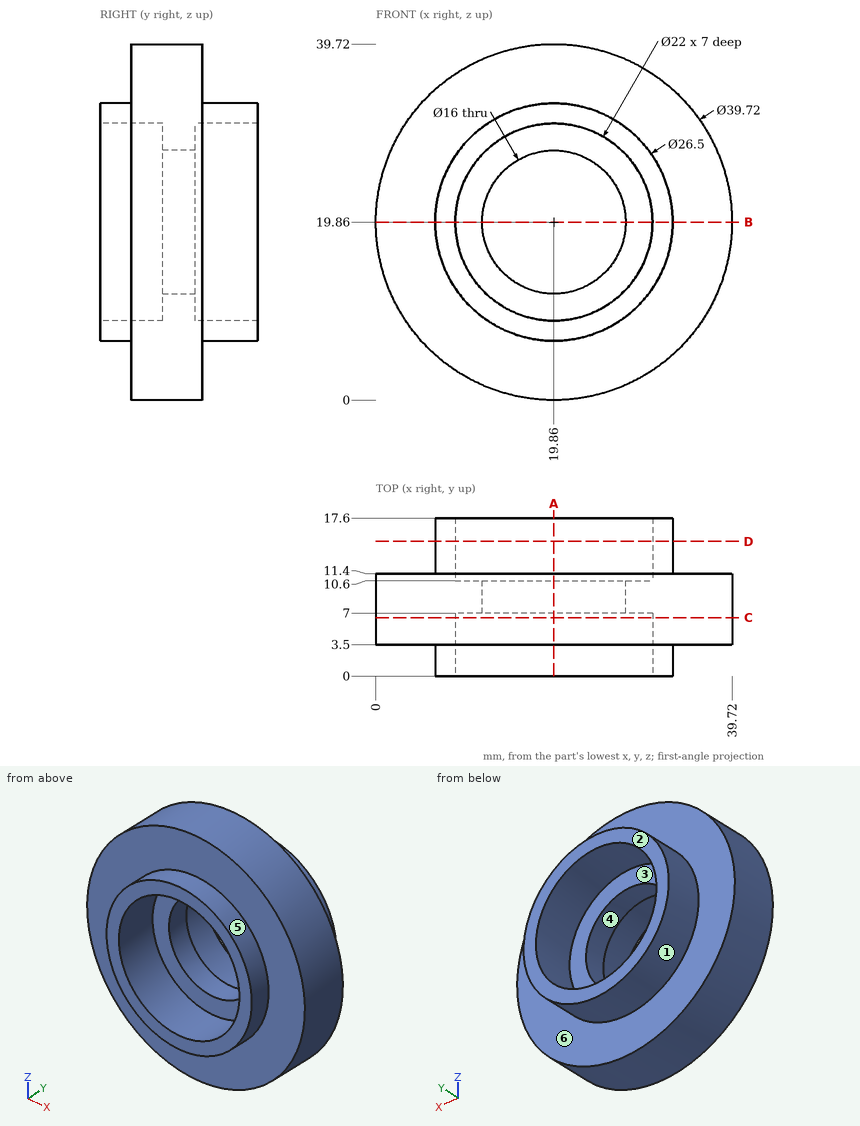
Part print with two shaded views. Sizes in mm from the minimum x, y, z corner. A direction names the side the tool comes from. Coordinates: 2 decimals unless noted, no trailing zeros. Write each loop counter-clockwise with the first axis right and the second up, starting at its lowest first coordinate (ties: lowest second). Pieces come first, ordered by that corner, then holes. Notation, with made-up numbers: (-30, 89.5) - (-23, 89.5) arc R18 cw to (-23, 101.5) - close; hole circle Ø1 at (32, 21). An arc over 180 degrees is marked (long way). Use a Markdown table: item, result. Add a question column.
Item 1: 3-axis set-ups, long thin cutter, end or side, ignore diameter. For the marked faces 4, 5 and 6: which of +Z, -Z, +X, -X, +Y, -Y reach the whole face in a straight line?
Item 2: Band-saw the part on D-D, the plane y = 15. Write the cut outline in (x, z), and give its area (3 significant figures).
Item 3: Band-saw the part on A-A, the plane x = 19.86. Write the cut outline in (y, z).
Item 4: Two-plate mould, pull along Z, no slides. Class the marked faces 1, 2 and 3: pulls with the +Z half, pulls with the -Z half, needs draft (parallel to the pull), parting line crosses it, or undercut.
Item 5: Drop flat-ended pins along their axis: pin 1 (5 mm diameter, centred on x = 24, z = 31.5, fed in from -Y); pin 2 (4 mm diameter, centred on x = 13.5, y = 14.5, fed in from +Z); pin 3 (12 mm diameter, centred on x = 21, z = 24, fed in from -Y); pin 4 (18.5 mm diameter, centred on x = 19.86, z = 19.86, fed in from +Y). Give the stop position or say it passes through.
Item 6: Band-saw the part on B-B, the plane z = 19.86. Write the cut outline in (x, y), and give its area (3 significant figures).
Item 7: Band-saw the part on C-C, the plane y = 6.5. Write the cut outline in (x, z), and give its area (3 significant figures).
Item 8: Drill centre lines: line 1 along X through (y, z) = (13.5, 19.86); line 2 along X through (y, z) = (8.95, 19.86); line 3 along Z through (x, y) = (12, 14.5). Where is each one in solid material? Low to high.
A:
| question | item | result |
|---|---|---|
| 1 | face 4 | +Y, -Y |
| 1 | face 5 | -Y |
| 1 | face 6 | +Y |
| 2 | outline | circle Ø26.5 at (19.86, 19.86); hole circle Ø22 at (19.86, 19.86) |
| 2 | area | 171 mm² |
| 3 | outline | (0, 6.61) - (3.5, 6.61) - (3.5, 0) - (11.4, 0) - (11.4, 6.61) - (17.6, 6.61) - (17.6, 8.86) - (10.6, 8.86) - (10.6, 11.86) - (7, 11.86) - (7, 8.86) - (0, 8.86) - close; (0, 30.86) - (7, 30.86) - (7, 27.86) - (10.6, 27.86) - (10.6, 30.86) - (17.6, 30.86) - (17.6, 33.11) - (11.4, 33.11) - (11.4, 39.72) - (3.5, 39.72) - (3.5, 33.11) - (0, 33.11) - close |
| 4 | face 1 | parting line crosses it |
| 4 | face 2 | needs draft |
| 4 | face 3 | undercut |
| 5 | pin 1 | stops at y = 0 |
| 5 | pin 2 | stops at z = 32.37 |
| 5 | pin 3 | stops at y = 7 |
| 5 | pin 4 | stops at y = 10.6 |
| 6 | outline | (0, 3.5) - (6.61, 3.5) - (6.61, 0) - (8.86, 0) - (8.86, 7) - (11.86, 7) - (11.86, 10.6) - (8.86, 10.6) - (8.86, 17.6) - (6.61, 17.6) - (6.61, 11.4) - (0, 11.4) - close; (27.86, 7) - (30.86, 7) - (30.86, 0) - (33.11, 0) - (33.11, 3.5) - (39.72, 3.5) - (39.72, 11.4) - (33.11, 11.4) - (33.11, 17.6) - (30.86, 17.6) - (30.86, 10.6) - (27.86, 10.6) - close |
| 6 | area | 205 mm² |
| 7 | outline | circle Ø39.72 at (19.86, 19.86); hole circle Ø22 at (19.86, 19.86) |
| 7 | area | 859 mm² |
| 8 | line 1 | x = 6.61 to 8.86, 30.86 to 33.11 |
| 8 | line 2 | x = 0 to 11.86, 27.86 to 39.72 |
| 8 | line 3 | z = 9.19 to 12.16, 27.56 to 30.53 |
